from build123d import *

# Parameters (mm, degrees)
SKETCH_1_W          = 80
SKETCH_1_H          = 130
SKETCH_1_R          = 4.5
EXTRUDE_1_DEPTH     = 4
CHAMFER_1_SIZE      = 25
CUT_EXTRUDE_1_DEPTH = 5
SKETCH_4_R          = 2.15
CUT_EXTRUDE_2_DEPTH = 4
SKETCH_5_R          = 1.6
CUT_EXTRUDE_3_DEPTH = 4


with BuildPart() as part:
    # 草图1 → 凸台-拉伸1 (new body)
    with BuildSketch(Plane.XY):
        with Locations((0, 21)):
            Rectangle(SKETCH_1_W, SKETCH_1_H)
        with Locations((0, -29)):
            Circle(SKETCH_1_R, mode=Mode.SUBTRACT)
    extrude(amount=-EXTRUDE_1_DEPTH)

    # 倒角1
    chamfer_1_edges = [part.edges().sort_by_distance(p)[0] for p in [
        (40, -44, -2),
        (-40, -44, -2),
    ]]
    chamfer(chamfer_1_edges, length=CHAMFER_1_SIZE)

    # 草图3 → 切除-拉伸1 (cut)
    with BuildSketch(Plane(origin=(0, 0, -4), x_dir=(-1, 0, 0), z_dir=(0, 0, -1))):
        with BuildLine():
            ThreePointArc((-27, 58.07), (-29.121320344, 57.191320344), (-30, 55.07))
            Line((-30, 55.07), (-30, 44))
            ThreePointArc((-30, 44), (-29.121320344, 41.878679656), (-27, 41))
            Line((-27, 41), (27, 41))
            ThreePointArc((27, 41), (29.121320344, 41.878679656), (30, 44))
            Line((30, 44), (30, 55.07))
            ThreePointArc((30, 55.07), (29.121320344, 57.191320344), (27, 58.07))
            Line((27, 58.07), (-17.606738259, 58.07))
            Line((-17.606738259, 58.07), (-27, 58.07))
        make_face()
        with BuildLine():
            Line((-27, 26), (27, 26))
            ThreePointArc((27, 26), (29.121320344, 25.121320344), (30, 23))
            Line((30, 23), (30, -11))
            ThreePointArc((30, -11), (29.121320344, -13.121320344), (27, -14))
            Line((27, -14), (-27, -14))
            ThreePointArc((-27, -14), (-29.121320344, -13.121320344), (-30, -11))
            Line((-30, -11), (-30, 23))
            ThreePointArc((-30, 23), (-29.121320344, 25.121320344), (-27, 26))
        make_face()
    extrude(amount=-CUT_EXTRUDE_1_DEPTH, mode=Mode.SUBTRACT)

    # 草图4 → 切除-拉伸2 (cut)
    with BuildSketch(Plane(origin=(0, 0, -4), x_dir=(-1, 0, 0), z_dir=(0, 0, -1))):
        with Locations((-34, 32)):
            Circle(SKETCH_4_R)
        with Locations((34, 32)):
            Circle(SKETCH_4_R)
    extrude(amount=-CUT_EXTRUDE_2_DEPTH, mode=Mode.SUBTRACT)

    # 草图5 → 切除-拉伸3 (cut)
    with BuildSketch(Plane(origin=(0, 0, -4), x_dir=(-1, 0, 0), z_dir=(0, 0, -1))):
        with Locations((34, 75)):
            Circle(SKETCH_5_R)
        with Locations((22, 75)):
            Circle(SKETCH_5_R)
        with Locations((-22, 75)):
            Circle(SKETCH_5_R)
        with Locations((-34, 75)):
            Circle(SKETCH_5_R)
        with Locations((34, 62)):
            Circle(SKETCH_5_R)
        with Locations((22, 62)):
            Circle(SKETCH_5_R)
        with Locations((-22, 62)):
            Circle(SKETCH_5_R)
        with Locations((-34, 62)):
            Circle(SKETCH_5_R)
    extrude(amount=-CUT_EXTRUDE_3_DEPTH, mode=Mode.SUBTRACT)


solid = part.part
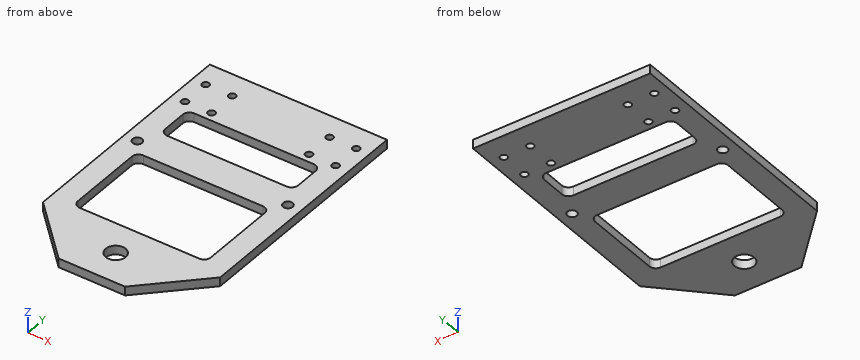
CAD build for the part. Positions are in the model's coordinates, mm. Coordinates: 2 decimals unless noted, no trailing zeros. Order: outer loops, then holes, each group sorted by start corner. A loop starts at its lowest first (then second) coordinate and runs counter-clockwise, first axis right, second up. Notation, with made-up numbers: (76.5, -11.75) -> (134.5, -11.75) arc R19 ccw to (134.5, 7.25) -> close; hole circle Ø8 at (-13, -11). An arc over 180 degrees is marked (long way). Answer in a Markdown table with one row per item.
1) Flat gauge pins, fed straight in: P1, Ø3.5, axis at x = -22, y = 62, coming from the -Z side; P2, Ø10, axis at x = 8.5, y = 18.5, coming from the +Z side. Where does each tip first touch, or does it go through?
Check values:
| item | result |
|---|---|
| P1 | z = -4 |
| P2 | through |
2) Band-saw the part on C-C (y = -29). List the corners of the cut face in (x, z).
Check values:
| item | result |
|---|---|
| outline | (-30, -4) -> (-4.5, -4) -> (-4.5, 0) -> (-30, 0) -> close; (4.5, -4) -> (30, -4) -> (30, 0) -> (4.5, 0) -> close |
3) Band-saw the part on A-A (y = 75). List the corners of the cut face in (x, z).
Check values:
| item | result |
|---|---|
| outline | (-40, -4) -> (-35.6, -4) -> (-35.6, 0) -> (-40, 0) -> close; (-32.4, -4) -> (-23.6, -4) -> (-23.6, 0) -> (-32.4, 0) -> close; (-20.4, -4) -> (20.4, -4) -> (20.4, 0) -> (-20.4, 0) -> close; (23.6, -4) -> (32.4, -4) -> (32.4, 0) -> (23.6, 0) -> close; (35.6, -4) -> (40, -4) -> (40, 0) -> (35.6, 0) -> close |
4) Band-saw the part on D-D (z = -2.65). Give the number of separate pieces and of enclosed holes in the cut face, and give its area (3 significant figures).
Check values:
| item | result |
|---|---|
| separate pieces | 1 |
| enclosed holes | 13 |
| area | 6,210 mm2 |
5) Drill centre lines: line 1 (Y direction, x = -7.5, z = -2.85); line 2 (X direction, y = 75, z = -2.7); line 3 (Y direction, x = 22, z = -1.55). Where is each one in solid material? Low to high.
Check values:
| item | result |
|---|---|
| line 1 | -44 to -14, 26 to 41, 58.07 to 86 |
| line 2 | -40 to -35.6, -32.4 to -23.6, -20.4 to 20.4, 23.6 to 32.4, 35.6 to 40 |
| line 3 | -37 to -14, 26 to 41, 58.07 to 60.4, 63.6 to 73.4, 76.6 to 86 |
6) Band-saw the part on B-B (x = -16.5). List the corners of the cut face in (y, z), and give its area (3 significant figures).
Check values:
| item | result |
|---|---|
| outline | (-42.5, -4) -> (-14, -4) -> (-14, 0) -> (-42.5, 0) -> close; (26, -4) -> (41, -4) -> (41, 0) -> (26, 0) -> close; (58.07, -4) -> (86, -4) -> (86, 0) -> (58.07, 0) -> close |
| area | 286 mm2 |
